```python
from build123d import *

# Parameters (mm, degrees)
BOSS_EXTRUDE1_DEPTH = 12.7
CUT_EXTRUDE1_DEPTH  = 6.35
CHAMFER1_SIZE       = 1.27


with BuildPart() as part:
    # Sketch1 → Boss-Extrude1 (new body)
    with BuildSketch(Plane.XY):
        Polygon((-80.433333333, 19.05), (-80.433333333, -6.35), (80.433333333, -6.35), (80.433333333, 19.05), (67.733333333, 19.05), (67.733333333, 6.35), (-67.733333333, 6.35), (-67.733333333, 19.05), align=None)
    extrude(amount=BOSS_EXTRUDE1_DEPTH)

    # Sketch2 → Cut-Extrude1 (cut)
    with BuildSketch(Plane(origin=(0, 19.05, 0), x_dir=(1, 0, 0), z_dir=(0, 1, 0))):
        Polygon((-78.573461394, -6.35), (-74.083333333, -1.859871939), (-69.593205273, -6.35), (-74.083333333, -10.840128061), align=None)
        Polygon((69.593205273, -6.35), (74.083333333, -1.859871939), (78.573461394, -6.35), (74.083333333, -10.840128061), align=None)
    extrude(amount=-CUT_EXTRUDE1_DEPTH, mode=Mode.SUBTRACT)

    # Chamfer1
    chamfer1_edges = [part.edges().sort_by_distance(p)[0] for p in [
        (-76.328397364, 12.7, 8.59506403),
        (-76.328397364, 12.7, 4.10493597),
        (-71.838269303, 12.7, 4.10493597),
        (-71.838269303, 12.7, 8.59506403),
        (-76.328397364, 19.05, 8.59506403),
        (-71.838269303, 19.05, 8.59506403),
        (-71.838269303, 19.05, 4.10493597),
        (-76.328397364, 19.05, 4.10493597),
        (71.838269303, 12.7, 8.59506403),
        (71.838269303, 12.7, 4.10493597),
        (76.328397364, 12.7, 4.10493597),
        (76.328397364, 12.7, 8.59506403),
        (71.838269303, 19.05, 8.59506403),
        (76.328397364, 19.05, 8.59506403),
        (76.328397364, 19.05, 4.10493597),
        (71.838269303, 19.05, 4.10493597),
    ]]
    chamfer(chamfer1_edges, length=CHAMFER1_SIZE)


solid = part.part
```
Work out the finished part from the listing and answer in its coordinate system (mm). A direction names the side the tool comes from. Give positions to 0.01 mm unless a question says otherwise; leave off trailing zeros. Loops run counter-clockwise (first coordinate to the right, second up) from the corner with the lowest first, then second, coordinate; pieces in that order, holes last. Notation, with made-up numbers: (49, -38.5) - (100, -38.5) arc R24 cw to (100, -10.5) - close; hole circle Ø9 at (-39, 27.5). An arc over 180 degrees is marked (long way). One line per question, with ' | ' between items.
(1) Each of these flat-tipped pins is pushed along its axis until it touches: pin 1 Ø1.5 at (x, z) = (50, 9) entering from +Y; pin 2 Ø2.5 at (x, z) = (-75, 7) entering from +Y; pin 3 Ø2.5 at (x, z) = (74, 6) entering from +Y. Where does it stop, or does it pass through?
Recorded:
pin 1: stops at y = 6.35 | pin 2: stops at y = 13.15 | pin 3: stops at y = 12.7
(2) The part is cut by section A-A (y = 11.25). Write down the section's boundary in (x, z), then the cut area to 3 significant figures.
Recorded:
outline: (-80.43, 0) - (-67.73, 0) - (-67.73, 12.7) - (-80.43, 12.7) - close; (67.73, 0) - (80.43, 0) - (80.43, 12.7) - (67.73, 12.7) - close | area: 323 mm²
(3) The part is cut by section B-B (x = -48). Write down the section's boundary in (y, z).
Recorded:
outline: (-6.35, 0) - (6.35, 0) - (6.35, 12.7) - (-6.35, 12.7) - close
(4) A tool of negligible diameter and unlimited length cuts with its end or side. For faces 4 (the face through (-1, 1, 12.7)), 5 (the face through (1, 6.35, 6)), 6 (the face through (-76.36, 15.902, 4.136)), from which of +Z, -Z, +X, -X, +Y, -Y can it reach the whole face along a straight path? Write none if from no direction.
Recorded:
face 4: +Z, +X, -X, +Y, -Y | face 5: +Z, -Z, +Y | face 6: +Y
(5) The mould has two halves that part along X. Classify faces 1 (the face through (-75.905, 13.326, 4.592)), 2 (the face through (-78, 19.05, 9)), 3 (the face through (80.433, 6, 6)): +X half, -X half, draft (parallel to the pull), parting line (faces both ways), or undercut.
Recorded:
face 1: undercut | face 2: draft | face 3: +X half
(6) Straight lines are drawn through the part: probe 1 along X at (y, z) = (11, 6.25); probe 2 along X at (y, z) = (17.25, 7.25); probe 3 along X at (y, z) = (16.75, 8). For each, find the intervals that lie inside material, in ascending order.
Recorded:
probe 1: x = -80.43 to -67.73, 67.73 to 80.43 | probe 2: x = -80.43 to -77.67, -70.49 to -67.73, 67.73 to 70.49, 77.67 to 80.43 | probe 3: x = -80.43 to -76.92, -71.24 to -67.73, 67.73 to 71.24, 76.92 to 80.43
